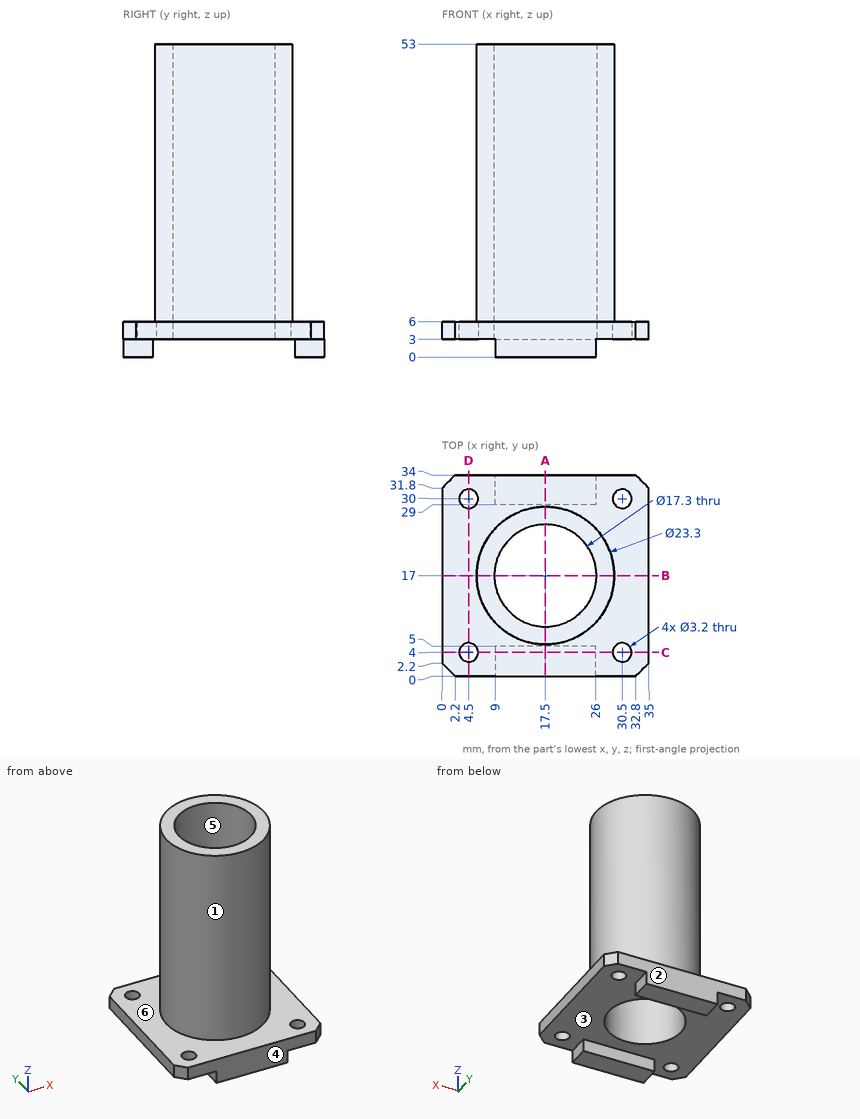
Geometry check sheet. Reference: drawing and pictorial views, mm from the part's lowest x, y, z. A direction names the side the tool comes from. Round coordinates to 2 decimals unless told otherwise and drop trailing zeros. Loops run counter-clockwise (first coordinate to the right, second up) from the corner with the lowest first, then second, coordinate; pieces in that order, holes last. Notation, with made-up numbers: (-29.75, 19.25) - (-0.75, 19.25) arc R17 ccw to (-0.75, 26.25) - close; hole circle Ø5 at (-29, 82). An arc over 180 degrees is marked (long way). Use a Markdown table: item, result. Add a question column.
1. Section check D-D, the plane x = 4.5. Record the boundary of the cut face in (y, z).
2. Release check for a two-part mould opening along Y. For the marked faces 3, 4, 5 and 6 record: released by +Y, released by -Y, zero draft, split by the parting line, or undercut.
3. Section check B-B, the plane y = 17. Record the boundary of the cut face in (x, z).
4. Access from +Z, -Z, +X, -X, +Y, -Y to the whole of each face (thin tool, end or side, straight path). Record for the marked faces 1 and 2.
5. Gauge pin test, flat ends, axial feed: pin 1 (4 mm diameter, centred on x = 30.5, y = 30, fed in from -Z); pin 2 (2.5 mm diameter, centred on y = 3, z = 1.5, fed in from -X); pin 3 (2.5 mm diameter, centred on y = 32, z = 2, fed in from -X); pin 4 (1.5 mm diameter, centred on y = 3.5, z = 2, fed in from +X). Record the tip position at first contact, or that the pin passes through.
6. Section check A-A, the plane x = 17.5. Record the boundary of the cut face in (y, z), plus the area to 3 significant figures.
7. Section check C-C, the plane y = 4. Record the boundary of the cut face in (x, z), plus the area to 3 significant figures.
8. Thickness scan on probe 1 along X at (y, z) = (30, 4); probe 2 along Y at (x, z) = (30.5, 4.35); probe 3 along Y at (x, z) = (4, 4). Record the ranges inside material, lowest first. Write a range as [from, to].
Checks:
| question | item | result |
|---|---|---|
| 1 | outline | (0, 3) - (2.4, 3) - (2.4, 6) - (0, 6) - close; (5.6, 3) - (28.4, 3) - (28.4, 6) - (5.6, 6) - close; (31.6, 3) - (34, 3) - (34, 6) - (31.6, 6) - close |
| 2 | face 3 | undercut |
| 2 | face 4 | released by -Y |
| 2 | face 5 | undercut |
| 2 | face 6 | zero draft |
| 3 | outline | (0, 3) - (8.85, 3) - (8.85, 53) - (5.85, 53) - (5.85, 6) - (0, 6) - close; (26.15, 3) - (35, 3) - (35, 6) - (29.15, 6) - (29.15, 53) - (26.15, 53) - close |
| 4 | face 1 | +Z |
| 4 | face 2 | +Z, -Z, +X, -X, +Y |
| 5 | pin 1 | stops at z = 3 |
| 5 | pin 2 | stops at x = 9 |
| 5 | pin 3 | stops at x = 0 |
| 5 | pin 4 | stops at x = 26 |
| 6 | outline | (0, 0) - (5, 0) - (5, 3) - (8.35, 3) - (8.35, 53) - (5.35, 53) - (5.35, 6) - (0, 6) - close; (25.65, 3) - (29, 3) - (29, 0) - (34, 0) - (34, 6) - (28.65, 6) - (28.65, 53) - (25.65, 53) - close |
| 6 | area | 362 mm^2 |
| 7 | outline | (0, 3) - (2.9, 3) - (2.9, 6) - (0, 6) - close; (6.1, 3) - (9, 3) - (9, 0) - (26, 0) - (26, 3) - (28.9, 3) - (28.9, 6) - (6.1, 6) - close; (32.1, 3) - (35, 3) - (35, 6) - (32.1, 6) - close |
| 7 | area | 137 mm^2 |
| 8 | probe 1 | x = [0, 2.9], [6.1, 28.9], [32.1, 35] |
| 8 | probe 2 | y = [0, 2.4], [5.6, 28.4], [31.6, 34] |
| 8 | probe 3 | y = [0, 2.48], [5.52, 28.48], [31.52, 34] |
